Could you check a few things on this drawing? It's one solid part, dimensions in mm from its lowest x, y, z. Round coordinates to 2 decimals unless told otherwise and drop trailing zeros. Write each loop counter-clockwise with the first axis right and the second up, starting at its lowest first coordinate (ties: lowest second). Pieces come first, ordered by that corner, then holes. Notation, with made-up numbers: (-9, 46.5) -> (-1, 46.5) arc R12 cw to (-1, 58.5) -> close; hole circle Ø11 at (88.25, 87). An arc over 180 degrees is marked (long way). Return JSON: item names as keys, results as strings.
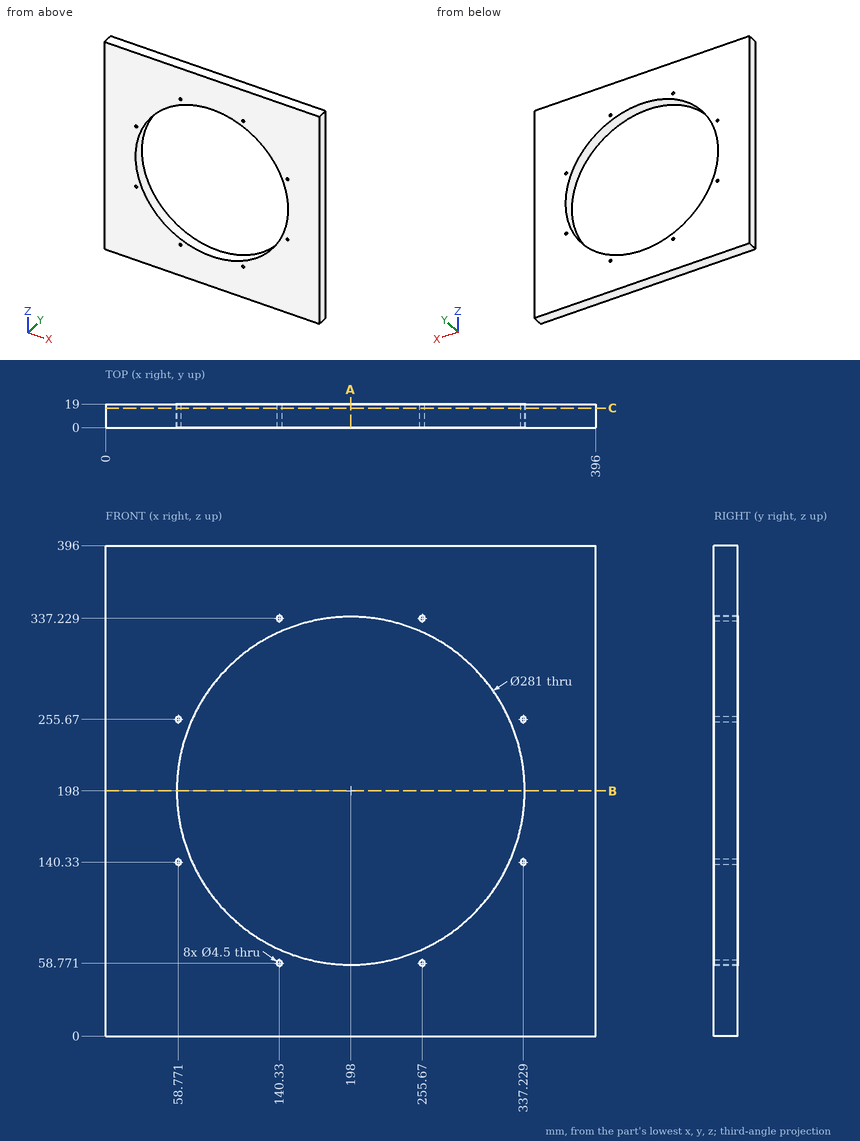
1) I want a section at C-C, the plane y = 15.75. Count the separate pieces of the cut face and the enclosed holes in it, and give its area (3 significant figures).
Return value:
{"separate pieces": "1", "enclosed holes": "9", "area": "94,700 mm²"}
2) I want a section at B-B, the plane z = 198. Please give me the cut outline in (x, y), and give its area (4 significant figures).
Return value:
{"outline": "(0, 0) -> (57.5, 0) -> (57.5, 19) -> (0, 19) -> close; (338.5, 0) -> (396, 0) -> (396, 19) -> (338.5, 19) -> close", "area": "2,185 mm²"}
3) If I drill on probe 1 along X at (y, z) = (18.25, 229.5); probe 2 along Z at (x, y) = (144, 18.25); probe 3 along Z at (x, y) = (278, 1.5), over which ranges is the centre line in solid material (lowest first)? Write a range as [from, to].
Return value:
{"probe 1": "[0, 61.08], [334.92, 396]", "probe 2": "[0, 68.29], [327.71, 396]", "probe 3": "[0, 82.5], [313.5, 396]"}
4) I want a section at A-A, the plane x = 198. Please give me the cut outline in (y, z), and give its area (4 significant figures).
Return value:
{"outline": "(0, 0) -> (19, 0) -> (19, 57.5) -> (0, 57.5) -> close; (0, 338.5) -> (19, 338.5) -> (19, 396) -> (0, 396) -> close", "area": "2,185 mm²"}
